Autodesk Inventor part; units mm, degrees
ref_plane "YZ Plane" through (0, 0, 0) normal (1, 0, 0) x (0, 1, 0)
ref_plane "XZ Plane" through (0, 0, 0) normal (0, 1, 0) x (-1, 0, 0)
ref_plane "XY Plane" through (0, 0, 0) normal (0, 0, 1) x (1, 0, 0)
sketch "Sketch1" plane through (0, 0, 0) normal (1, 0, 0) x (0, 1, 0)
  line L0 (-66.675, -66.675) -> (66.675, -66.675)
  line L1 (66.675, -66.675) -> (66.675, 66.675)
  line L2 (66.675, 66.675) -> (-66.675, 66.675)
  line L3 (-66.675, 66.675) -> (-66.675, -66.675)
  line L4 (-66.675, -66.675) -> (66.675, 66.675) construction
  line L5 (66.675, -66.675) -> (-66.675, 66.675) construction
  point P0 (0, 0)
  dimension "d0" = 133.35
  dimension "d1" = 133.35
extrude "Extrusion1" add sketch "Sketch1" along normal blind 6.35
sketch "Sketch2" plane through (6.35, 0, 0) normal (1, 0, 0) x (0, 0, -1)
  line L0 (56.5875, -56.5875) -> (-56.5875, -56.5875)
  line L1 (-56.5875, -56.5875) -> (-56.5875, 56.5875)
  line L2 (-56.5875, 56.5875) -> (56.5875, 56.5875)
  line L3 (56.5875, 56.5875) -> (56.5875, -56.5875)
  line L4 (56.5875, -56.5875) -> (-56.5875, 56.5875) construction
  line L5 (-56.5875, -56.5875) -> (56.5875, 56.5875) construction
  point P0 (0, 0)
  dimension "d4" = 113.175
  dimension "d5" = 113.175
extrude "Extrusion2" cut sketch "Sketch2" against normal blind 3.175
sketch "Sketch3" plane through (3.175, 0, 0) normal (1, 0, 0) x (0, 0, -1)
  line L0 (56.5875, -56.5875) -> (-56.5875, -56.5875)
  line L1 (56.5875, 56.5875) -> (56.5875, -56.5875)
  line L2 (-56.5875, 56.5875) -> (56.5875, 56.5875)
  line L3 (-56.5875, -56.5875) -> (-56.5875, 56.5875)
  line L4 (-53.4125, 53.4125) -> (53.4125, 53.4125)
  line L5 (53.4125, 53.4125) -> (53.4125, -53.4125)
  line L6 (53.4125, -53.4125) -> (-53.4125, -53.4125)
  line L7 (-53.4125, -53.4125) -> (-53.4125, 53.4125)
  point P0 (0, 0)
  dimension "d8" = 3.175
extrude "Extrusion3" cut sketch "Sketch3" against normal through all contours L4 L5 L6 L7
equation "\"d0\" = width + internalAcrylicThickness"
equation "\"d1\" = height + internalAcrylicThickness"
equation "\"d2\" = internalAcrylicThickness"
equation "\"d4\" = aerogelHeight + aerogelClearence"
equation "\"d5\" = aerogelWidth + aerogelClearence"
equation "\"d6\" = 0.5 * internalAcrylicThickness"
equation "\"d8\" = aerogelClearence"
equation "\"d9\" = 0.5 * internalAcrylicThickness"
equation "\"frameAcrylicThickness\" = 9.525"
equation "\"internalAcrylicThickness\" = 6.35"
equation "\"aerogelWidth\" = 110"
equation "\"aerogelHeight\" = 110"
equation "\"height\" = 127"
equation "\"width\" = 127"
equation "\"depth\" = 273.05"
equation "\"mirrorAngle\" = 5deg"
equation "\"detectorWidth\" = 52"
equation "\"detectorHeight\" = 52"
equation "\"mirrorThickness\" = 3.175"
equation "\"fresnelThickness\" = 0.1"
equation "\"focalLength\" = 76.2"
equation "\"ior\" = 1.49"
equation "\"centerThickness\" = 1.524"
equation "\"fresnelAngle\" = 90deg"
equation "\"fresnelEffectiveDiameter\" = 152.4"
equation "\"oRingWidth\" = 1.5875"
equation "\"sensorHolderDepth\" = 19.05"
equation "\"aerogelClearence\" = 3.175"
equation "\"backplanePostionOffsett\" = 12.7"
equation "\"backplaneHoleOffsett\" = 6.35"
equation "\"backplanePCBHeight\" = 76.2"
equation "\"backplanePCBWidth\" = 76.2"
equation "\"moduleSlotClearence\" = 0.79375"
properties part number "aerogelHolder" material "ABS Plastic"
Could you check a few things on this model? Use its own coordinates, in mm. A direction names the side the tool comes from. Give positions to 0.01 mm unless a question says otherwise; leave off trailing zeros. Write each loop counter-clockwise with the first axis right and the second up, starting at its lowest first coordinate (ties: lowest second). Pieces come first, ordered by that corner, then holes. Notation, with made-up numbers: (16.5, -8.75) -> (71.5, -8.75) arc R18 ccw to (71.5, 8.25) -> close; hole circle Ø4 at (52.25, 23). An arc over 180 degrees is marked (long way). Write each question's results on one line, items separated by ' | '. Start each with the question number.
Q1. We'd pull the mould along Z, two halves only. Please class faces 1 (the face through (5, 56.588, 1)), 2 (the face through (3, 1, 66.675)), 3 (the face through (3, -66.675, 1)), 4 (the face through (3, -1, -66.675)): +Z half, -Z half, draft (parallel to the pull), parting line (faces both ways), or undercut.
Q2. I need wall thicknesses on probe 1 along Y at (x, z) = (5.5, -27) (1 decimal); probe 2 along Y at (x, z) = (1.25, 2) (1 decimal). Which ranges of each line are inside material? Lowest first, please.
Q3. Which directions (+Z, -Z, +X, -X, +Y, -Y) give clear straight access to the entire face, cutting with the end or side of a thin tool? Please do faces 5 (the face through (2, -1, 53.412)), 6 (the face through (3, 66.675, -1)), 7 (the face through (5, 1, -56.588)).
Q4. Suppose I cut it at C-C, the plane x = 1.5. List the corners of the cut face in (y, z) for me (1 decimal).
Outcome:
1) face 1: undercut | face 2: +Z half | face 3: draft | face 4: -Z half
2) probe 1: -66.7 to -56.6, 56.6 to 66.7 | probe 2: -66.7 to -53.4, 53.4 to 66.7
3) face 5: +X, -X | face 6: +Z, -Z, +X, -X, +Y | face 7: +X
4) outline: (-66.7, -66.7) -> (66.7, -66.7) -> (66.7, 66.7) -> (-66.7, 66.7) -> close; hole (-53.4, -53.4) -> (53.4, -53.4) -> (53.4, 53.4) -> (-53.4, 53.4) -> close
